```python
from build123d import *

# Parameters (mm, degrees)
SKETCH_1_W        = 8
SKETCH_1_H        = 8
FOAM_PAD_DEPTH    = 2.3
SENSOR_START      = 2.3
SKETCH_2_W        = 9
SKETCH_2_H        = 9
SENSOR_PCB_DEPTH  = 1.1
LENS_START        = 3.4
SKETCH_3_W        = 8.5
SKETCH_3_H        = 8.5
LENS_HOLDER_DEPTH = 3.5
LENS_START_2      = 6.9
SKETCH_4_R        = 3.25
LENS_BARREL_DEPTH = 1.8
LENS_START_3      = 8.7
SKETCH_5_R        = 3.45
LENS_RING_DEPTH   = 0.3
LENS_START_4      = 9
SKETCH_6_R        = 1.7
LENS_GLASS_DEPTH  = 0.2


with BuildPart() as part:
    # 草圖1 → foam pad (new body)
    with BuildSketch(Plane.XY):
        with Locations((30, -25)):
            Rectangle(SKETCH_1_W, SKETCH_1_H)
    extrude(amount=FOAM_PAD_DEPTH)

    # 草圖2 → sensor PCB (add)
    with BuildSketch(Plane.XY.offset(SENSOR_START)):
        with Locations((30, -25)):
            Rectangle(SKETCH_2_W, SKETCH_2_H)
    extrude(amount=SENSOR_PCB_DEPTH)

    # 草圖3 → lens holder (add)
    with BuildSketch(Plane.XY.offset(LENS_START)):
        with Locations((30, -25)):
            Rectangle(SKETCH_3_W, SKETCH_3_H)
    extrude(amount=LENS_HOLDER_DEPTH)

    # 草圖4 → lens barrel (add)
    with BuildSketch(Plane.XY.offset(LENS_START_2)):
        with Locations((30, -25)):
            Circle(SKETCH_4_R)
    extrude(amount=LENS_BARREL_DEPTH)

    # 草圖5 → lens ring (add)
    with BuildSketch(Plane.XY.offset(LENS_START_3)):
        with Locations((30, -25)):
            Circle(SKETCH_5_R)
    extrude(amount=LENS_RING_DEPTH)

    # 草圖6 → lens glass (add)
    with BuildSketch(Plane.XY.offset(LENS_START_4)):
        with Locations((30, -25)):
            Circle(SKETCH_6_R)
    extrude(amount=LENS_GLASS_DEPTH)


solid = part.part
```
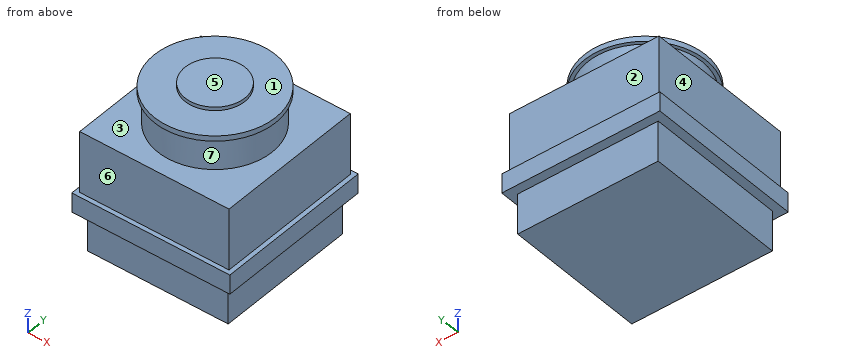
Work out the finished part from the listing and answer in its coordinate system (mm). Face numbers are marked on the shaded views. A direction names the side the tool comes from. Give positions to 0.01 mm unless a question says otherwise; leave off trailing zeros. Loops run counter-clockwise (first coordinate to the right, second up) from the corner with the lowest first, then second, coordinate; pieces in that order, holes last. Notation, with made-up numbers: (19.5, 82.5) - (33.5, 82.5) arc R20 cw to (33.5, 89.5) - close; hole circle Ø11 at (34, 85.25). An arc over 180 degrees is marked (long way). Use CSV: the item, a comma, the result in double quotes. Start each with the question number.
(1) Determine the mould class of the marked faces 5, 6 and 7 for opening direction Z: released by +Z, released by -Z, zero draft, split by the parting line, or undercut.
(2) Find section A-A, the plane x = 30. Determine the outline of the cut face in (y, z), plus the area to 3 significant figures.
(3) Each of these flat-tipped pins is pushed along its axis until it touches: pin 1 (2 mm diameter, centred on y = -26, z = 1, fed in from -X); pin 2 (3 mm diameter, centred on y = -25.5, z = 5.5, fed in from -X); pin 3 (2.5 mm diameter, centred on x = 30.5, z = 1, fed in from +Y). Where does it stop, or does it pass through?
(4) A tool of negligible diameter and unlimited length cuts with its end or side. For the marked faces 1, 2, 3 and 4, from which of +Z, -Z, +X, -X, +Y, -Y can it reach the whole face along a straight path? Write none if from no direction.
(5) Find the intervals of material crossed by L1, parallel to Y at x = 30.25, z = 2; L2, parallel to Y at x = 30, z = 8.25; L3, parallel to X at y = -25.25, z = 1.75, in increasing order.
(6) Find section B-B, the plane y = -25. Determine the outline of the cut face in (x, z).
(7) Find section C-C, the plane z = 5.25. Determine the outline of the cut face in (x, y).
(8) Find section D-D, the plane y = -22.5. Determine the outline of the cut face in (x, z).
Results found:
1,face 5,"released by +Z"
1,face 6,"zero draft"
1,face 7,"undercut"
2,outline,"(-29.5, 2.3) - (-29, 2.3) - (-29, 0) - (-21, 0) - (-21, 2.3) - (-20.5, 2.3) - (-20.5, 3.4) - (-20.75, 3.4) - (-20.75, 6.9) - (-21.75, 6.9) - (-21.75, 8.7) - (-21.55, 8.7) - (-21.55, 9) - (-23.3, 9) - (-23.3, 9.2) - (-26.7, 9.2) - (-26.7, 9) - (-28.45, 9) - (-28.45, 8.7) - (-28.25, 8.7) - (-28.25, 6.9) - (-29.25, 6.9) - (-29.25, 3.4) - (-29.5, 3.4) - close"
2,area,"72.5 mm^2"
3,pin 1,"x = 26"
3,pin 2,"x = 25.75"
3,pin 3,"y = -21"
4,face 1,"+Z"
4,face 2,"+Z, +X, -X, +Y"
4,face 3,"none"
4,face 4,"+Z, -X, +Y, -Y"
5,L1,"-29 to -21"
5,L2,"-28.25 to -21.75"
5,L3,"26 to 34"
6,outline,"(25.5, 2.3) - (26, 2.3) - (26, 0) - (34, 0) - (34, 2.3) - (34.5, 2.3) - (34.5, 3.4) - (34.25, 3.4) - (34.25, 6.9) - (33.25, 6.9) - (33.25, 8.7) - (33.45, 8.7) - (33.45, 9) - (31.7, 9) - (31.7, 9.2) - (28.3, 9.2) - (28.3, 9) - (26.55, 9) - (26.55, 8.7) - (26.75, 8.7) - (26.75, 6.9) - (25.75, 6.9) - (25.75, 3.4) - (25.5, 3.4) - close"
7,outline,"(25.75, -29.25) - (34.25, -29.25) - (34.25, -20.75) - (25.75, -20.75) - close"
8,outline,"(25.5, 2.3) - (26, 2.3) - (26, 0) - (34, 0) - (34, 2.3) - (34.5, 2.3) - (34.5, 3.4) - (34.25, 3.4) - (34.25, 6.9) - (32.08, 6.9) - (32.08, 8.7) - (32.38, 8.7) - (32.38, 9) - (27.62, 9) - (27.62, 8.7) - (27.92, 8.7) - (27.92, 6.9) - (25.75, 6.9) - (25.75, 3.4) - (25.5, 3.4) - close"
